Can you work these out from the drawing? Everything is in mm from the part's minimum corner. Coordinates: 2 decimals unless noted, no trailing zeros. Order: outer loops, then holes, each group sorted by start corner. A loop starts at its lowest first (then second) coordinate and runs counter-clockwise, first axis right, second up. Notation, with made-up numbers: (1.5, -12.5) -> (37.5, -12.5) arc R18 ccw to (37.5, -7.5) -> close; hole circle Ø9 at (-39.75, 68.25). An arc over 180 degrees is marked (long way). Use a Markdown table: item, result. Add a question column.
1) If I drill on L1, parallel to X at y = 4.5, z = 81.65; L2, parallel to Z at x = 80.5, y = 1.25; L3, parallel to Z at x = 58, y = 8, over which ranges is the centre line in solid material (lowest first)? Write a range as [from, to].
2) If we section it at A-A (y = 5): Give the number of separate pieces and of enclosed holes in the cut face, plus the area to 3 significant figures.
3) Will these pins go through, and if not, where does the flat tip stop? pin 1 Ø5 at (y, z) = (6.5, 50) entering from +X (1 decimal); pin 2 Ø0.9 at (x, y) = (6, 3.5) entering from +Z; pin 3 Ø1 at (x, y) = (71.5, 8.5) entering from +Z (1 decimal).
4) If we section it at B-B (z = 89.5): Write out the boundary of the cut face in (x, y).
5) If we section it at C-C (x = 100.5): Write out the boundary of the cut face in (y, z) (1 decimal).
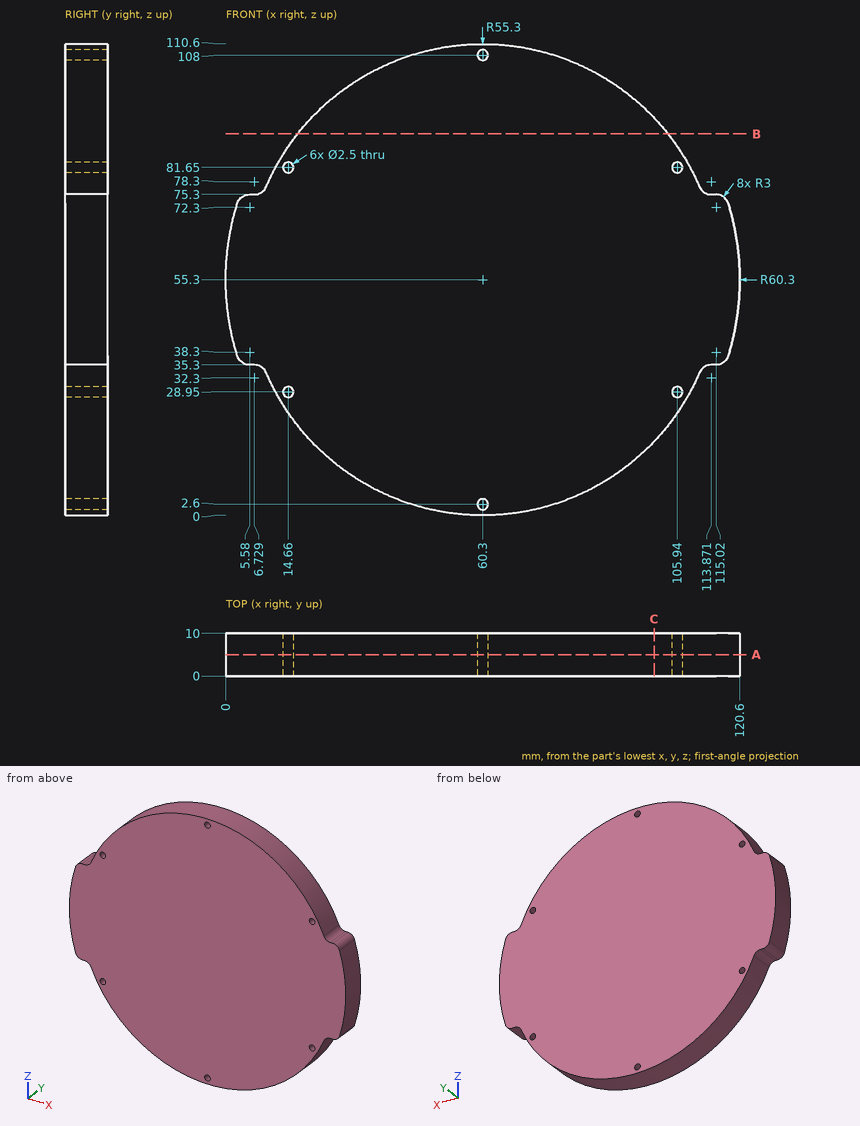
Answer sheet:
| question | item | result |
|---|---|---|
| 1 | L1 | [11.68, 13.41], [15.91, 104.69], [107.19, 108.92] |
| 1 | L2 | [3.82, 106.78] |
| 1 | L3 | [0.05, 110.55] |
| 2 | separate pieces | 1 |
| 2 | enclosed holes | 6 |
| 2 | area | 9,990 mm2 |
| 3 | pin 1 | x = 120.5 |
| 3 | pin 2 | z = 75.3 |
| 3 | pin 3 | z = 109.6 |
| 4 | outline | (16.84, 0) -> (103.76, 0) -> (103.76, 10) -> (16.84, 10) -> close |
| 5 | outline | (0, 17.3) -> (10, 17.3) -> (10, 93.3) -> (0, 93.3) -> close |
